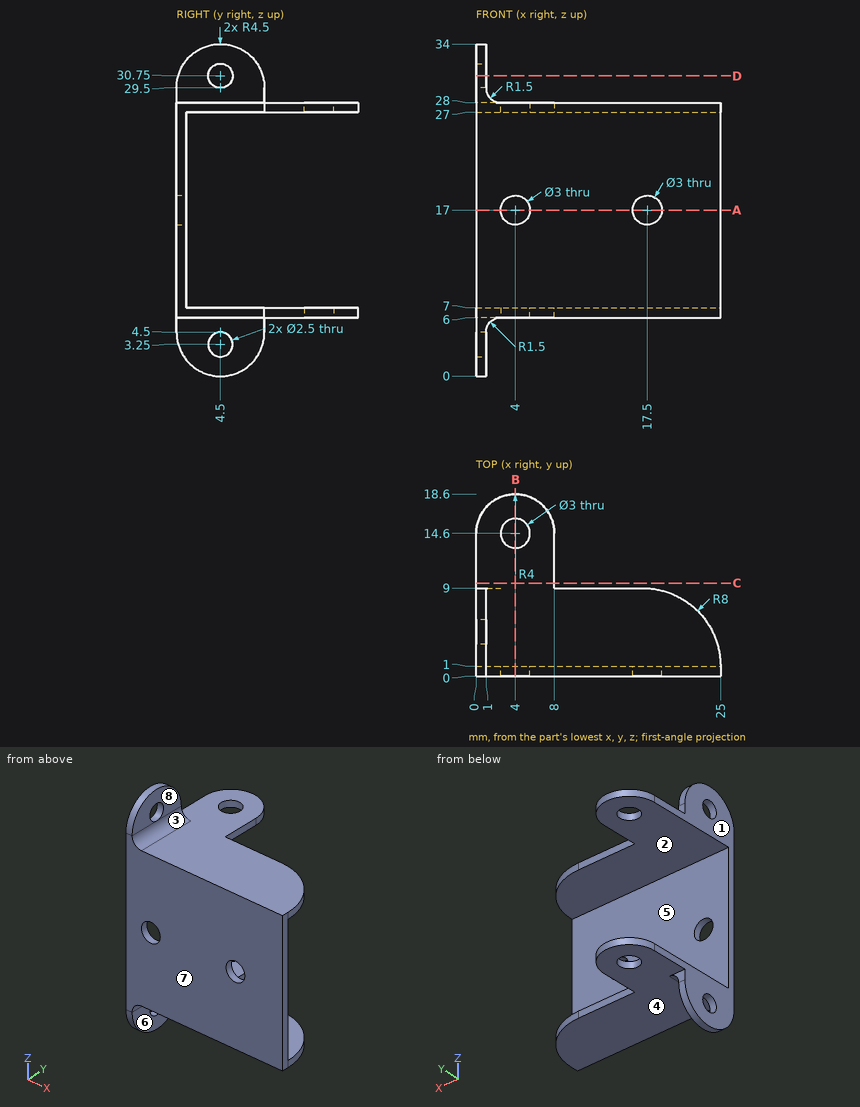
The drawing under review shows one solid part. Ordinate dimensions are in mm from its lowest x, y, z. A direction names the side the tool comes from. Coordinates: 2 decimals unless noted, no trailing zeros. Write each loop counter-clockwise with the first axis right and the second up, starting at its lowest first coordinate (ties: lowest second). Pieces come first, ordered by that corner, then holes.
1) Machinability: for the marked faces 5, 6, 7 and 8, which of the approach directions +Z, -Z, +X, -X, +Y, -Y give a long, thin tool a straight path to every point of the face, cutting with its end or side? Answer none if there is none.
2) Add section A-A (z = 17). Write out the cut boundary in (x, y), plus the area to 3 significant figures.
3) Add section C-C (y = 9.5). Write out the cut boundary in (x, z), plus the area to 3 significant figures.
4) To check wall thickness, follow L1, parallel to X at y = 0.3, z = 17; L2, parallel to Z at x = 0.2, y = 4.5; L3, parallel to Z at x = 12.25, y = 1.25. State the ranges of each line that lie inside material, in increasing order.
5) Mouldability with a two-part tool opening along Z and no side actions: class the marked faces 1, 2, 3 and 4 as +Z half, -Z half, draft (parallel to the pull), parting line (faces both ways), or undercut.
6) Add section D-D (z = 30.75). Write out the cut boundary in (x, y), plus the area to 3 significant figures.
7) Add section B-B (x = 4). Write out the cut boundary in (y, z), plus the area to 3 significant figures.
8) Insertion check: pin 1 (3 mm diameter, centred on x = 13, z = 20, fed in from +Y); pin 2 (3 mm diameter, centred on x = 12, y = 6, fed in from -Z); pin 3 (1.1 mm diameter, centred on y = 12.5, z = 27.5, fed in from +X); pin 4 (5 mm diameter, centred on x = 5, z = 19, fed in from -Y). Each pin has a flat end and moves straight along its axis. Give the tip position at first contact, or say it passes through.
Check result:
1. face 5: +X, -X, +Y
1. face 6: -Z, +X, +Y, -Y
1. face 7: +Z, -Z, +X, -X, -Y
1. face 8: +Z, +X, +Y, -Y
2. outline: (0, 0) - (2.5, 0) - (2.5, 1) - (0, 1) - close; (5.5, 0) - (16, 0) - (16, 1) - (5.5, 1) - close; (19, 0) - (25, 0) - (25, 1) - (19, 1) - close
2. area: 19.0 mm2
3. outline: (0, 6) - (8, 6) - (8, 7) - (0, 7) - close; (0, 27) - (8, 27) - (8, 28) - (0, 28) - close
3. area: 16.0 mm2
4. L1: x = 0 to 2.5, 5.5 to 16, 19 to 25
4. L2: z = 0 to 2, 4.5 to 7, 27 to 29.5, 32 to 34
4. L3: z = 6 to 7, 27 to 28
5. face 1: draft
5. face 2: undercut
5. face 3: +Z half
5. face 4: -Z half
6. outline: (0, 0.18) - (1, 0.18) - (1, 3.25) - (0, 3.25) - close; (0, 5.75) - (1, 5.75) - (1, 8.82) - (0, 8.82) - close
6. area: 6.15 mm2
7. outline: (0, 6) - (13.1, 6) - (13.1, 7) - (1, 7) - (1, 15.5) - (0, 15.5) - close; (0, 18.5) - (1, 18.5) - (1, 27) - (13.1, 27) - (13.1, 28) - (0, 28) - close; (16.1, 6) - (18.6, 6) - (18.6, 7) - (16.1, 7) - close; (16.1, 27) - (18.6, 27) - (18.6, 28) - (16.1, 28) - close
7. area: 48.2 mm2
8. pin 1: stops at y = 1
8. pin 2: stops at z = 6
8. pin 3: stops at x = 8
8. pin 4: stops at y = 0
